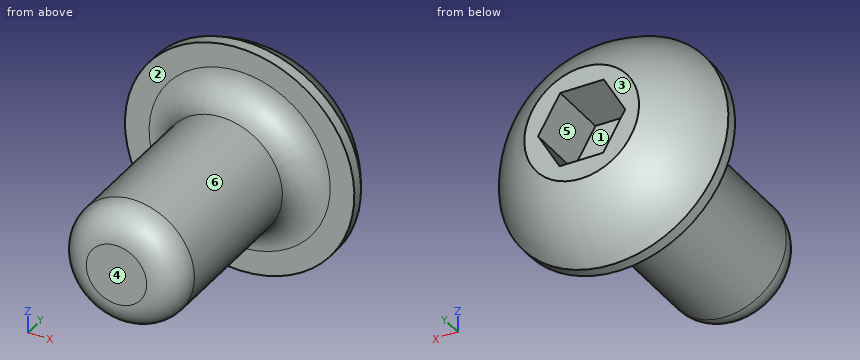
```python
from build123d import *

# Parameters (mm, degrees)
SKETCH1_R           = 2
BOSS_EXTRUDE1_DEPTH = 7
CUT_EXTRUDE1_DEPTH  = 2
FILLET1_R           = 1


with BuildPart() as part:
    # Sketch1 → Boss-Extrude1 (new body)
    with BuildSketch(Plane(origin=(0, 0, 0), x_dir=(1, 0, 0), z_dir=(0, 1, 0))):
        with Locations(Location((0, 0, 0), (0, 0, 270))):
            Circle(SKETCH1_R)
    extrude(amount=BOSS_EXTRUDE1_DEPTH)

    # Sketch2 → Revolve1 (revolve)
    with BuildSketch(Plane.XY, mode=Mode.PRIVATE) as revolve1_sk:
        with BuildLine():
            Line((0, 7), (3.8, 7))
            Line((3.8, 7), (3.8, 7.38))
            ThreePointArc((3.8, 7.38), (2.991926525, 8.438165054), (1.9, 9.2))
            Line((1.9, 9.2), (0, 9.2))
            Line((0, 9.2), (0, 7))
        make_face()
    revolve(revolve1_sk.sketch.rotate(Axis((0, 7, 0), (0, 1, 0)), 90), axis=Axis((0, 7, 0), (0, 1, 0)))

    # Sketch3 → Cut-Extrude1 (cut)
    with BuildSketch(Plane(origin=(0, 9.2, 0), x_dir=(1, 0, 0), z_dir=(0, 1, 0))):
        Polygon((-0.73360086, -1.243045901), (0.709708899, -1.256839931), (1.443309758, -0.01379403), (0.73360086, 1.243045901), (-0.709708899, 1.256839931), (-1.443309758, 0.01379403), align=None)
    extrude(amount=-CUT_EXTRUDE1_DEPTH, mode=Mode.SUBTRACT)

    # Fillet1
    fillet1_edges = [part.edges().sort_by_distance(p)[0] for p in [
        (0, 0, -2),
        (0, 7, -2),
    ]]
    fillet(fillet1_edges, radius=FILLET1_R)


solid = part.part
```
The listing builds one solid part. Answer for the finished solid, in the listing's coordinates (mm). Face numbers are marked on the shaded views. A direction names the side the tool comes from. Round coordinates to 2 decimals unless told otherwise and drop trailing zeros. Write each loop counter-clockwise with the first axis right and the second up, starting at its lowest first coordinate (ties: lowest second). Pieces come first, ordered by that corner, then holes. Notation, with made-up numbers: (78, 80) -> (85, 80) arc R25 cw to (85, 119) -> close; hole circle Ø9 at (-10, -30). An arc over 180 degrees is marked (long way). Write item = value, one per line.
1) Which of the six approach directions +Z, -Z, +X, -X, +Y, -Y give full straight-line access (tool end or side, diameter ignored) to the marked faces 1, 2 and 3?
Check values:
face_1 = +Y
face_2 = -Y
face_3 = +Z, -Z, +X, -X, +Y
2) Given pin 1 (1.5 mm diameter, centred on x = -1, z = 0, fed in from +Y); pin 2 (1 mm diameter, centred on y = 3.5, z = -1, fed in from +X); pin 3 (4 mm diameter, centred on x = -1.5, y = 3, fed in from +Z); pin 4 (1.3 mm diameter, centred on x = -0.5, z = 0, fed in from +Y), each flat-ended and moving along its own axis, determine where each tip first touches the part or whether it passes through.
Check values:
pin_1 = 9.2
pin_2 = 1.94
pin_3 = 2
pin_4 = 7.2
3) For a pull along Z with two mould halves and no side action, classify the marked faces 4, 5 and 6 as released by +Z, released by -Z, zero draft, split by the parting line, or undercut.
Check values:
face_4 = zero draft
face_5 = undercut
face_6 = split by the parting line
4) Section A-A on y = 5 is taken. Write down the section's boundary in (x, z).
Check values:
outline = circle Ø4 at (0, 0)
5) Straight lines are drawn through the part: line 1 along Y through (x, z) = (-0.25, 1); line 2 along Y through (x, z) = (1.25, -2.75); line 3 along Z through (x, y) = (1, 1.25). For each, find the intervals that lie inside material, in ascending order. Write a range as [from, to].
Check values:
line_1 = [0, 7.2]
line_2 = [7, 8.41]
line_3 = [-1.73, 1.73]
